Read the model definition and answer for the solid it produces. Units are mm, in the model's axes. A direction names the side the tool comes from. Coordinates: 2 decimals unless noted, no trailing zeros. Write each loop counter-clockwise with the first axis right and the second up, starting at its lowest first coordinate (ties: lowest second). Pieces come first, ordered by that corner, then holes. Notation, with made-up numbers: (30, -2) -> (71, -2) arc R19 cw to (71, 8) -> close; hole circle Ø1 at (16, -9.5). An arc over 180 degrees is marked (long way). Return JSON: item names as keys, results as strings.
from build123d import *

# Parameters (mm, degrees)
PAD_DEPTH       = 70
SKETCH001_W     = 11.887794
SKETCH001_H     = 46.78
POCKET_DEPTH    = 70.001
POCKET001_DEPTH = 30
SKETCH003_R     = 2.4
POCKET002_DEPTH = 15
POCKET003_DEPTH = 3.5
POCKET004_DEPTH = 9
SKETCH021_W     = 28
SKETCH021_H     = 53.161749
POCKET005_DEPTH = 10
SKETCH022_W     = 32
SKETCH022_H     = 58.660217
POCKET006_DEPTH = 28
POCKET007_DEPTH = 51
SKETCH008_W     = 19.05323
SKETCH008_H     = 10.69447
SKETCH008_W_2   = 35.750058
SKETCH008_H_2   = 36.172176
POCKET008_DEPTH = 45
SKETCH009_R     = 1.9
POCKET009_DEPTH = 5
SKETCH015_W     = 11
SKETCH015_H     = 38.184422
SKETCH015_W_2   = 19.881198
SKETCH015_H_2   = 10
PAD001_DEPTH    = 8
SKETCH011_R     = 1.9
POCKET010_DEPTH = 10
SKETCH010_R     = 1.6
POCKET011_DEPTH = 7
SKETCH017_R     = 3
POCKET012_DEPTH = 2
SKETCH013_R     = 1.9
POCKET013_DEPTH = 10
SKETCH014_W     = 10
SKETCH014_H     = 15
PAD002_DEPTH    = 18


with BuildPart() as part:
    # Sketch → Pad (new body)
    with BuildSketch(Plane.XY):
        Polygon((0, 0), (45, 0), (45, -50), (-28, -50), (-28, 0), align=None)
    extrude(amount=PAD_DEPTH)

    # Sketch001 (on Face7 of Pad) → Pocket (cut, through all)
    with BuildSketch(Plane.XY.offset(70)):
        with Locations((34.056103, -28.39)):
            Rectangle(SKETCH001_W, SKETCH001_H)
    extrude(amount=-POCKET_DEPTH, mode=Mode.SUBTRACT)

    # Sketch002 (on Face5 of Pocket) → Pocket001 (cut)
    with BuildSketch(Plane.XY.offset(70)):
        Polygon((30, -5), (30, -65.096024), (-40.783405, -65.096024), (-40.783405, 12.994774), (20, 12.994774), (20, -5), align=None)
    extrude(amount=-POCKET001_DEPTH, mode=Mode.SUBTRACT)

    # Sketch003 (on Face6 of Pocket001) → Pocket002 (cut)
    with BuildSketch(Plane.XY.offset(40)):
        with Locations((-22, -40)):
            Circle(SKETCH003_R)
        with Locations((22, -40)):
            Circle(SKETCH003_R)
    extrude(amount=-POCKET002_DEPTH, mode=Mode.SUBTRACT)

    # Sketch004 (on Face6 of Pocket002) → Pocket003 (cut)
    with BuildSketch(Plane.XY.offset(40)):
        with BuildLine():
            ThreePointArc((8.125, -40), (0, -31.875), (-8.125, -40))
            Line((-8.125, -59.24), (-8.125, -40))
            Line((8.125, -59.24), (-8.125, -59.24))
            Line((8.125, -40), (8.125, -59.24))
        make_face()
    extrude(amount=-POCKET003_DEPTH, mode=Mode.SUBTRACT)

    # Sketch018 → Pocket004 (cut)
    with BuildSketch(Plane.XY.offset(36.5)):
        with BuildLine():
            ThreePointArc((6.1, -40), (0, -33.9), (-6.1, -40))
            Line((-6.1, -40), (-6.1, -50))
            Line((6.1, -50), (-6.1, -50))
            Line((6.1, -40), (6.1, -50))
        make_face()
    extrude(amount=-POCKET004_DEPTH, mode=Mode.SUBTRACT)

    # Sketch021 (on Face9 of Pocket004) → Pocket005 (cut)
    with BuildSketch(Plane.XZ.offset(50)):
        with Locations((0, 16.83664)):
            Rectangle(SKETCH021_W, SKETCH021_H)
    extrude(amount=-POCKET005_DEPTH, mode=Mode.SUBTRACT)

    # Sketch022 (on Face13 of Pocket005) → Pocket006 (cut)
    with BuildSketch(Plane.XZ.offset(50)):
        with Locations((0, 1.369891)):
            Rectangle(SKETCH022_W, SKETCH022_H)
    extrude(amount=-POCKET006_DEPTH, mode=Mode.SUBTRACT)

    # Sketch023 (on Face9 of Pocket006) → Pocket007 (cut)
    with BuildSketch(Plane.XZ.offset(50)):
        Polygon((-38.33, 22), (6, 22), (24, -8), (-38.33, -8), align=None)
    extrude(amount=-POCKET007_DEPTH, mode=Mode.SUBTRACT)

    # Sketch008 (on Face14 of Pocket007) → Pocket008 (cut)
    with BuildSketch(Plane.XZ.offset(50)):
        with Locations((44.142395, 67.347235)):
            Rectangle(SKETCH008_W, SKETCH008_H)
        with Locations((52.797694, 0.913912)):
            Rectangle(SKETCH008_W_2, SKETCH008_H_2)
    extrude(amount=-POCKET008_DEPTH, mode=Mode.SUBTRACT)

    # Sketch009 (on Face3 of Pocket008) → Pocket009 (cut)
    with BuildSketch(Plane.YZ.offset(45)):
        with Locations((-44, 55)):
            Circle(SKETCH009_R)
        with Locations((-13, 24)):
            Circle(SKETCH009_R)
        with Locations((-13, 55)):
            Circle(SKETCH009_R)
        with Locations((-44, 24)):
            Circle(SKETCH009_R)
    extrude(amount=-POCKET009_DEPTH, mode=Mode.SUBTRACT)

    # Sketch015 (on Face26 of Pocket009) → Pad001 (join)
    with BuildSketch(Plane(origin=(-28, 0, 0), x_dir=(0, -1, 0), z_dir=(-1, 0, 0))):
        with Locations((13.5, 54.907789)):
            Rectangle(SKETCH015_W, SKETCH015_H)
        with Locations((52.059401, 30)):
            Rectangle(SKETCH015_W_2, SKETCH015_H_2)
    extrude(amount=-PAD001_DEPTH)

    # Sketch011 (on Face26 of Pad001) → Pocket010 (cut)
    with BuildSketch(Plane(origin=(-28, 0, 0), x_dir=(0, -1, 0), z_dir=(-1, 0, 0))):
        with Locations((56.5, 30)):
            Circle(SKETCH011_R)
        with Locations((13, 68.5)):
            Circle(SKETCH011_R)
    extrude(amount=-POCKET010_DEPTH, mode=Mode.SUBTRACT)

    # Sketch010 (on Face1 of Pocket010) → Pocket011 (cut)
    with BuildSketch(Plane(origin=(0, 0, 0), x_dir=(-1, 0, 0), z_dir=(0, 1, 0))):
        with Locations((-33, 5)):
            Circle(SKETCH010_R)
        with Locations((-40, 65)):
            Circle(SKETCH010_R)
        with Locations((-26, 65)):
            Circle(SKETCH010_R)
    extrude(amount=-POCKET011_DEPTH, mode=Mode.SUBTRACT)

    # Sketch017 (on Face31 of Pocket011) → Pocket012 (cut)
    with BuildSketch(Plane.XZ.offset(5)):
        with Locations((26, 65)):
            Circle(SKETCH017_R)
        with Locations((33, 5)):
            Circle(SKETCH017_R)
        with Locations((40, 65)):
            Circle(SKETCH017_R)
    extrude(amount=-POCKET012_DEPTH, mode=Mode.SUBTRACT)

    # Sketch013 (on Face40 of Pocket012) → Pocket013 (cut)
    with BuildSketch(Plane.XZ.offset(40)):
        with Locations((-11, 34)):
            Circle(SKETCH013_R)
        with Locations((11, 34)):
            Circle(SKETCH013_R)
    extrude(amount=-POCKET013_DEPTH, mode=Mode.SUBTRACT)

    # Sketch014 (on Face4 of Pocket013) → Pad002 (join)
    with BuildSketch(Plane.YZ.offset(45)):
        with Locations((-30, 32.5)):
            Rectangle(SKETCH014_W, SKETCH014_H)
    extrude(amount=-PAD002_DEPTH)


solid = part.part
1. The part is cut by section A-A (z = 65). Determine the outline of the cut face in (x, y), then the cut area to 3 significant figures.
Taken from the geometry:
{"outline": "(-28, -19) -> (-20, -19) -> (-20, -8) -> (-28, -8) -> close; (20, -5) -> (23, -5) -> (23, -3) -> (24.4, -3) -> (24.4, 0) -> (20, 0) -> close; (27.6, -3) -> (29, -3) -> (29, -5) -> (37, -5) -> (37, -3) -> (38.4, -3) -> (38.4, 0) -> (27.6, 0) -> close; (41.6, -3) -> (43, -3) -> (43, -5) -> (45, -5) -> (45, 0) -> (41.6, 0) -> close", "area": "170 mm2"}
2. The part is cut by section D-D (y = -56.5). Determine the outline of the cut face in (x, z), then the cut area to 3 significant figures.
Taken from the geometry:
{"outline": "(-28, 25) -> (-20, 25) -> (-20, 28.1) -> (-28, 28.1) -> close; (-28, 31.9) -> (-20, 31.9) -> (-20, 35) -> (-28, 35) -> close", "area": "49.6 mm2"}
3. Flat-ended cylindrical pins translate along their axes: pin 1 Ø1.5 at (x, y) = (43.5, -32) entering from +Z; pin 2 Ø8 at (x, y) = (-5.5, -36) entering from +Z; pin 3 Ø10 at (y, z) = (-10, 16.5) entering from -X; pin 4 Ø2.5 at (x, z) = (26, 65) entering from -Y. Find the tip coordinate at first contact, or state that the pin passes through.
Taken from the geometry:
{"pin 1": "stops at z = 62", "pin 2": "stops at z = 40", "pin 3": "stops at x = 6.3", "pin 4": "passes through"}
4. Consider L1, parallel to X at y = -1.7, z = 65; L2, parallel to X at y = -37, z = 29; L3, parallel to Z at x = 41, y = -13. Determine where each line is inside the solid, lowest interval first.
Taken from the geometry:
{"L1": "x = 20 to 24.4, 27.6 to 38.4, 41.6 to 45", "L2": "x = -28 to -16, 16 to 28.11, 40 to 45", "L3": "z = 19 to 22.1, 25.9 to 53.1, 56.9 to 62"}
5. A tool of negligible diameter and unlimited length cuts with its end or side. For faces 1 (the face through (-14, -45, 35)), 2 (the face through (-16, -36, 26)), 3 (the face through (42, -28, 62)), 4 (the face through (30, -4, 5)), 5 (the face through (0.179, -31.877, 38.274)), from which of +Z, -Z, +X, -X, +Y, -Y can it reach the whole face along a straight path? Write none if from no direction.
Taken from the geometry:
{"face 1": "+Z, -Z, -Y", "face 2": "-Z, -Y", "face 3": "+Z, +X, -Y", "face 4": "-Y", "face 5": "+Z, -Y"}
6. For a pull along Z with two mould halves and no side action, classify faces 6 (the face through (-24, -62, 30)), 7 (the face through (-15, -20, 22)), 8 (the face through (37.6, -4, 63.2)) as +Z half, -Z half, draft (parallel to the pull), parting line (faces both ways), or undercut.
Taken from the geometry:
{"face 6": "draft", "face 7": "-Z half", "face 8": "undercut"}
7. The part is cut by section B-B (x = 33). Determine the outline of the cut face in (y, z).
Taken from the geometry:
{"outline": "(-35, 25) -> (-25, 25) -> (-25, 40) -> (-35, 40) -> close; (-5, 0) -> (0, 0) -> (0, 3.4) -> (-3, 3.4) -> (-3, 2) -> (-5, 2) -> close; (-5, 8) -> (-3, 8) -> (-3, 6.6) -> (0, 6.6) -> (0, 70) -> (-5, 70) -> close"}
8. The part is cut by section C-C (z = 47.5). Determine the outline of the cut face in (x, y).
Taken from the geometry:
{"outline": "(-28, -19) -> (-20, -19) -> (-20, -8) -> (-28, -8) -> close; (20, -5) -> (40, -5) -> (40, -50) -> (45, -50) -> (45, 0) -> (20, 0) -> close"}
